Autodesk Inventor part; units mm, degrees
ref_plane "YZ Plane" through (0, 0, 0) normal (1, 0, 0) x (0, 1, 0)
ref_plane "XZ Plane" through (0, 0, 0) normal (0, 1, 0) x (-1, 0, 0)
ref_plane "XY Plane" through (0, 0, 0) normal (0, 0, 1) x (1, 0, 0)
sketch "Sketch1" plane through (0, 0, 0) normal (0, 0, 1) x (1, 0, 0)
  line L0 (0, -180) -> (0, -156)
  line L1 (0, -180) -> (-50.3388, -180)
  line L2 (-208, -30) -> (-157.6612, -30)
  line L3 (-208, -30) -> (-208, -54)
  line L4 (-208, -180) -> (-208, -156)
  line L5 (-157.6612, -180) -> (-208, -180)
  line L6 (15, -15) -> (-223, -15)
  line L7 (-223, -15) -> (-223, -195)
  line L8 (-223, -195) -> (15, -195)
  line L9 (15, -195) -> (15, -15)
  circle A0 centre (-24, -42) radius 4.1
  circle A1 centre (-24, -88) radius 4.1
  circle A2 centre (-24, -122) radius 4.1
  circle A3 centre (-24, -168) radius 4.1
  circle A4 centre (-184, -168) radius 4.1
  circle A5 centre (-184, -122) radius 4.1
  circle A6 centre (-184, -88) radius 4.1
  circle A7 centre (-184, -42) radius 4.1
  line L10 (0, -30) -> (0, -54)
  line L11 (-50.3388, -30) -> (0, -30)
  dimension "d0" = 15
  dimension "d2" = 15
  dimension "d3" = 15
extrude "Extrusion1" add sketch "Sketch1" along normal blind 15
fillet "Fillet1" radius 30 4 edges at (15, -15, 7.5) (-223, -15, 7.5) (-223, -195, 7.5) (15, -195, 7.5)
sketch "Sketch2" plane through (0, 0, 15) normal (0, 0, 1) x (1, 0, 0)
  line L0 (-223, -45) -> (-223, -165) construction
  line L1 (-223, -105) -> (15, -105) construction
  line L2 (15, -165) -> (15, -45) construction
  line L3 (-193, -195) -> (-15, -195) construction
  line L4 (-104, -195) -> (-104, -15) construction
  line L5 (-15, -15) -> (-193, -15) construction
  point P0 (0, 0)
properties part number "front_plate_Z"
For this review, take the finished solid that the model builds, in its own axes (mm). Round coordinates to 2 decimals unless told otherwise and drop trailing zeros. Order: outer loops, then holes, each group sorted by start corner. A loop starts at its lowest first (then second) coordinate and runs counter-clockwise, first axis right, second up. Notation, with made-up numbers: (37.25, 54.25) -> (87.25, 54.25) arc R12 ccw to (87.25, 77.25) -> close; hole circle Ø10 at (-9, 47.25). An arc over 180 degrees is marked (long way). Put each result on its own line as item: value.
Q1. For probe 1 along Y at (x, z) = (-184, 11.25); probe 2 along X at (y, z) = (-29, 9); probe 3 along Y at (x, z) = (-13, 8.25), list the stretches that pass through material, from the lowest coordinate up. Write a range as [from, to].
Check result:
probe 1: [-195, -172.1], [-163.9, -126.1], [-117.9, -92.1], [-83.9, -46.1], [-37.9, -15]
probe 2: [-218.38, 10.38]
probe 3: [-194.93, -15.07]
Q2. Add section C-C on z = 7.5. State how many separate pieces and enclosed holes the cut face has, plus the area to 3 significant figures.
Check result:
separate pieces: 1
enclosed holes: 8
area: 41,600 mm2
Q3. Add section D-D on y = -42. Write out the cut boundary in (x, z).
Check result:
outline: (-222.85, 0) -> (-188.1, 0) -> (-188.1, 15) -> (-222.85, 15) -> close; (-179.9, 0) -> (-28.1, 0) -> (-28.1, 15) -> (-179.9, 15) -> close; (-19.9, 0) -> (14.85, 0) -> (14.85, 15) -> (-19.9, 15) -> close
Q4. Add section B-B on x = -24. Write out the cut boundary in (y, z), plus the area to 3 significant figures.
Check result:
outline: (-195, 0) -> (-172.1, 0) -> (-172.1, 15) -> (-195, 15) -> close; (-163.9, 0) -> (-126.1, 0) -> (-126.1, 15) -> (-163.9, 15) -> close; (-117.9, 0) -> (-92.1, 0) -> (-92.1, 15) -> (-117.9, 15) -> close; (-83.9, 0) -> (-46.1, 0) -> (-46.1, 15) -> (-83.9, 15) -> close; (-37.9, 0) -> (-15, 0) -> (-15, 15) -> (-37.9, 15) -> close
area: 2,210 mm2
Q5. Mouldability with a two-part tool opening along X and no side actions: class faces 1 (the cylindrical face through (-187.022, -124.771, 7.395)), 2 (the flat face through (-103, -15, 7)), 3 (the cylindrical face through (6.445, -24.021, 7.605)), 4 (the flat face through (-223, -104, 7)) as pulls with the +X half, pulls with the -X half, needs draft (parallel to the pull), parting line crosses it, or undercut.
Check result:
face 1: undercut
face 2: needs draft
face 3: pulls with the +X half
face 4: pulls with the -X half
Q6. Insertion check: pin 1 Ø7.5 at (x, y) = (-24, -168) entering from +Z; pin 2 Ø2 at (y, z) = (-38, 7.5) entering from -X; pin 3 Ø1 at (y, z) = (-40.5, 6.5) entering from -X. Each pin has a flat end and moves straight along its axis. Give the tip position at first contact, or say it passes through.
Check result:
pin 1: through
pin 2: x = -222.39
pin 3: x = -222.73
Q7. Add section A-A on y = -122. Write out the cut boundary in (x, z), plus the area to 3 significant figures.
Check result:
outline: (-223, 0) -> (-188.1, 0) -> (-188.1, 15) -> (-223, 15) -> close; (-179.9, 0) -> (-28.1, 0) -> (-28.1, 15) -> (-179.9, 15) -> close; (-19.9, 0) -> (15, 0) -> (15, 15) -> (-19.9, 15) -> close
area: 3,320 mm2
